```python
from build123d import *

# Parameters (mm, degrees)
BOSS_EXTRUDE1_DEPTH      = 6.2865
BOSS_EXTRUDE1_DEPTH_BACK = 6.2865
SKETCH1_R                = 6
BOSS_EXTRUDE2_DEPTH      = 2.2865
BOSS_EXTRUDE2_DEPTH_BACK = 2.2865
SKETCH2_R                = 6
SKETCH2_R_2              = 4.9


with BuildPart() as part:
    # Sketch1 → Boss-Extrude1 (new, two sides: drawn at the far end of the back side and taken through both)
    with BuildSketch(Plane(origin=(0, 0, 0), x_dir=(1, 0, 0), z_dir=(0, 1, 0)).offset(-BOSS_EXTRUDE1_DEPTH_BACK)):
        Polygon((-3.592850725, 6.223), (-7.18570145, 0), (-3.592850725, -6.223), (3.592850725, -6.223), (7.18570145, 0), (3.592850725, 6.223), align=None)
        with Locations(Location((0, 0, 0), (0, 0, 270))):
            Circle(SKETCH1_R, mode=Mode.SUBTRACT)
    extrude(amount=BOSS_EXTRUDE1_DEPTH + BOSS_EXTRUDE1_DEPTH_BACK)

    # Sketch2 → Boss-Extrude2 (add, two sides: drawn at the far end of the back side and taken through both)
    with BuildSketch(Plane(origin=(0, 0, 0), x_dir=(1, 0, 0), z_dir=(0, 1, 0)).offset(-BOSS_EXTRUDE2_DEPTH_BACK)):
        with Locations(Location((0, 0, 0), (0, 0, 270))):
            Circle(SKETCH2_R)
        with Locations(Location((0, 0, 0), (0, 0, 270))):
            Circle(SKETCH2_R_2, mode=Mode.SUBTRACT)
    extrude(amount=BOSS_EXTRUDE2_DEPTH + BOSS_EXTRUDE2_DEPTH_BACK)


solid = part.part
```
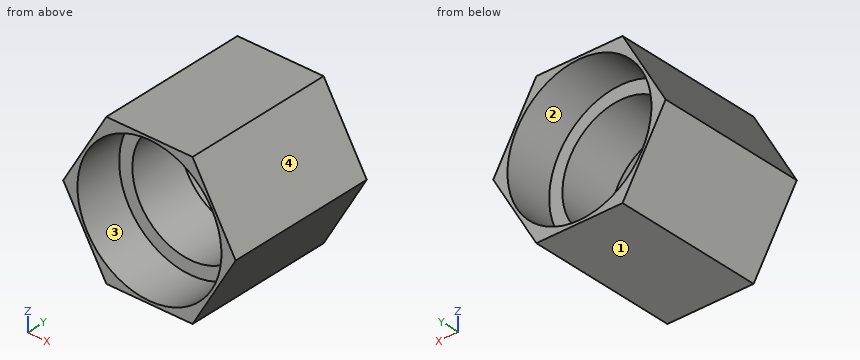
Here's how the part is built. I have some questions about the finished solid (model axes, mm). Face numbers are marked on the shaded views. Coordinates: 2 decimals unless noted, no trailing zeros. Loops run counter-clockwise (first coordinate to the right, second up) from the corner with the lowest first, then second, coordinate; pieces in that order, holes last. Notation, with made-up numbers: (-37.75, 10) - (10.25, 10) arc R21 ccw to (10.25, 14) - close; hole circle Ø10 at (-14, 1.5). An arc over 180 degrees is marked (long way). Answer as CSV lines item,"result".
Q1. If we section it at A-A, the plane x = 0: Write out the boundary of the cut face in (y, z).
Response:
outline,"(-6.29, -6.22) - (6.29, -6.22) - (6.29, -6) - (2.29, -6) - (2.29, -4.9) - (-2.29, -4.9) - (-2.29, -6) - (-6.29, -6) - close; (-6.29, 6) - (-2.29, 6) - (-2.29, 4.9) - (2.29, 4.9) - (2.29, 6) - (6.29, 6) - (6.29, 6.22) - (-6.29, 6.22) - close"
Q2. If we section it at D-D, the plane y = -4.5: Write out the boundary of the cut face in (x, z).
Response:
outline,"(-7.19, 0) - (-3.59, -6.22) - (3.59, -6.22) - (7.19, 0) - (3.59, 6.22) - (-3.59, 6.22) - close; hole circle Ø12 at (0, 0)"
Q3. If I drill on L1, parallel to Z at x = -4, y = 0.75; L2, parallel to X at y = 3.75, z = -1.75; L3, parallel to X at y = 3.25, z = -1.25, over which ranges is the centre line in solid material (lowest first)? Write a range as [from, to].
Response:
L1,"[-5.52, -2.83], [2.83, 5.52]"
L2,"[-6.18, -5.74], [5.74, 6.18]"
L3,"[-6.46, -5.87], [5.87, 6.46]"
Q4. We'd pull the mould along X, two halves only. Please class the marked faces 1, 2, 3 and 4: pulls with the +X half, pulls with the -X half, needs draft (parallel to the pull), parting line crosses it, or undercut.
Response:
face 1,"needs draft"
face 2,"undercut"
face 3,"undercut"
face 4,"pulls with the +X half"
Q5. If we section it at C-C, the plane z = -3.25: Write out the boundary of the cut face in (x, y).
Response:
outline,"(-5.31, -6.29) - (-5.04, -6.29) - (-5.04, -2.29) - (-3.67, -2.29) - (-3.67, 2.29) - (-5.04, 2.29) - (-5.04, 6.29) - (-5.31, 6.29) - close; (3.67, -2.29) - (5.04, -2.29) - (5.04, -6.29) - (5.31, -6.29) - (5.31, 6.29) - (5.04, 6.29) - (5.04, 2.29) - (3.67, 2.29) - close"
Q6. If we section it at B-B, the plane y = 0: Write out the boundary of the cut face in (x, z), and give its area (3 significant figures).
Response:
outline,"(-7.19, 0) - (-3.59, -6.22) - (3.59, -6.22) - (7.19, 0) - (3.59, 6.22) - (-3.59, 6.22) - close; hole circle Ø9.8 at (0, 0)"
area,"58.7 mm2"
Q7. For pin 1 (4 mm diameter, centred on x = -2, z = 1, fed in from +Y); pin 2 (3 mm diameter, centred on y = 1.5, z = 2.5, fed in from +X); pin 3 (3 mm diameter, centred on y = 0.5, z = -2, fed in from +X); pin 4 (4 mm diameter, centred on y = 2, z = 4, fed in from -X), each with a flat end and sliding along its axis, tell me the tip position at first contact or that it passes through.
Response:
pin 1,"through"
pin 2,"x = 6.61"
pin 3,"x = 6.9"
pin 4,"x = -6.03"
